Here's how the part is built. I have some questions about the finished solid (model axes, mm). A direction names the side the tool comes from. Round coordinates to 2 decimals unless told otherwise and drop trailing zeros. Order: outer loops, then holes, each group sorted by start corner. A loop starts at its lowest first (then second) coordinate and runs counter-clockwise, first axis right, second up. Notation, with made-up numbers: (41.25, -8) - (47.25, -8) arc R21 cw to (47.25, 29) - close; hole circle Ø5 at (20, 83). An arc over 180 degrees is marked (long way). Answer as a JSON object with one key per item and string values.
```python
from build123d import *

# Parameters (mm, degrees)
BOSS_EXTRUDE1_START                                 = 12.7
SKETCH1_W                                           = 108.839
SKETCH1_H                                           = 266.7
BOSS_EXTRUDE1_DEPTH                                 = 12.7
CBORE_FOR_8_BINDING_HEAD_MACHINE_SCREW1_D           = 4.9149
CBORE_FOR_8_BINDING_HEAD_MACHINE_SCREW1_CBORE_D     = 9.525
CBORE_FOR_8_BINDING_HEAD_MACHINE_SCREW1_CBORE_DEPTH = 2.667
SKETCH4_W                                           = 71.374
SKETCH4_H                                           = 223.52
CUT_EXTRUDE1_DEPTH                                  = 9.525
SKETCH6_R                                           = 2.38125
SKETCH8_W                                           = 12.7
SKETCH8_H                                           = 12.7
CUT_EXTRUDE3_DEPTH                                  = 9.525


with BuildPart() as part:
    # Sketch1 → Boss-Extrude1 (new body)
    with BuildSketch(Plane(origin=(0, 0, 0), x_dir=(1, 0, 0), z_dir=(0, 1, 0)).offset(BOSS_EXTRUDE1_START)):
        with Locations((91.6305, 133.35)):
            Rectangle(SKETCH1_W, SKETCH1_H)
    extrude(amount=BOSS_EXTRUDE1_DEPTH)

    # CBORE for #8 Binding Head Machine Screw1 (through all)
    with Locations(Plane(origin=(0, 25.4, 0), x_dir=(1, 0, 0), z_dir=(0, 1, 0))):
        with Locations((139.7, 6.35), (139.7, 260.35), (43.561, 6.35), (43.561, 260.35), (139.7, 133.35)):
            CounterBoreHole(CBORE_FOR_8_BINDING_HEAD_MACHINE_SCREW1_D / 2, CBORE_FOR_8_BINDING_HEAD_MACHINE_SCREW1_CBORE_D / 2, CBORE_FOR_8_BINDING_HEAD_MACHINE_SCREW1_CBORE_DEPTH)

    # Sketch4 → Cut-Extrude1 (cut)
    with BuildSketch(Plane(origin=(0, 12.7, 0), x_dir=(-1, 0, 0), z_dir=(0, -1, 0))):
        with Locations((-79.248, 130.175)):
            Rectangle(SKETCH4_W, SKETCH4_H)
    extrude(amount=-CUT_EXTRUDE1_DEPTH, mode=Mode.SUBTRACT)

    # Cut-Sweep1: sweep along a path in Sketch5
    with BuildLine(Plane.XZ.offset(-12.7)) as cut_sweep1_path:
        Line((114.935, -196.215), (120.015, -196.215))
        Line((120.015, -196.215), (120.015, -234.315))
        Line((120.015, -234.315), (128.905, -234.315))
        Line((128.905, -234.315), (128.905, -158.115))
        Line((128.905, -158.115), (137.795, -158.115))
        Line((137.795, -158.115), (137.795, -234.315))
        Line((137.795, -234.315), (146.05, -234.315))
    # Sketch6 → Cut-Sweep1 (sweep, cut)
    with BuildSketch(Plane(origin=(146.05, 0, 0), x_dir=(0, 0, -1), z_dir=(1, 0, 0))):
        with Locations((234.315, 12.7)):
            Circle(SKETCH6_R)
    sweep(path=cut_sweep1_path.line, transition=Transition.RIGHT, mode=Mode.SUBTRACT)

    # Sketch8 → Cut-Extrude3 (cut)
    with BuildSketch(Plane.XZ.offset(-12.7)):
        with Locations((121.285, -62.865)):
            Rectangle(SKETCH8_W, SKETCH8_H)
        with Locations((89.535, -248.285)):
            Rectangle(SKETCH8_W, SKETCH8_H)
    extrude(amount=-CUT_EXTRUDE3_DEPTH, mode=Mode.SUBTRACT)


solid = part.part
```
1. Imagine slicing it at B-B (y = 17.75). List the corners of the cut face in (x, z) for me (3 decimals), plus the area to 3 significant figures.
Responses:
{"outline": "(37.211, -266.7) - (146.05, -266.7) - (146.05, 0) - (37.211, 0) - close; hole circle Ø4.915 at (43.561, -260.35); hole circle Ø4.915 at (43.561, -6.35); hole (43.561, -241.935) - (83.185, -241.935) - (83.185, -254.635) - (95.885, -254.635) - (95.885, -241.935) - (114.935, -241.935) - (114.935, -69.215) - (127.635, -69.215) - (127.635, -56.515) - (114.935, -56.515) - (114.935, -18.415) - (43.561, -18.415) - close; hole circle Ø4.915 at (139.7, -260.35); hole circle Ø4.915 at (139.7, -133.35); hole circle Ø4.915 at (139.7, -6.35)", "area": "12,700 mm2"}
2. For faces 1 (the face through (142, 22.733, -258)), 2 (the face through (124.56, 14.92, -235.18)), 3 (the face through (142.155, 17.646, -6.458)), which set-ups out of +Z, -Z, +X, -X, +Y, -Y let a thin tool reach every point of the face, with its end or its side?
Responses:
{"face 1": "+Y", "face 2": "-Y", "face 3": "+Y, -Y"}
3. If I drill on L1, parallel to X at y = 24, z = -260.35; L2, parallel to Z at x = 139.7, y = 24.85; L3, parallel to X at y = 16.5, z = -33.5 (3 decimals), over which ranges is the centre line in solid material (lowest first)? Write a range as [from, to].
Responses:
{"L1": "[37.21, 38.8], [48.32, 134.94], [144.46, 146.05]", "L2": "[-266.7, -265.11], [-255.59, -138.11], [-128.59, -11.11], [-1.59, 0]", "L3": "[37.211, 43.561], [114.935, 146.05]"}
4. Thinking about a two-plate mould opening in Z: for faces 4 (the face through (91, 19, 0)), 5 (the face through (137.74, 15.08, -196.78)), which applies, pulls with the +Z half, pulls with the -Z half, needs draft (parallel to the pull), parting line crosses it, or undercut?
Responses:
{"face 4": "pulls with the +Z half", "face 5": "undercut"}
5. Imagine slicing it at D-D (x = 60). List the corners of the cut face in (y, z) for me (3 decimals), plus the area to 3 significant figures.
Responses:
{"outline": "(12.7, -266.7) - (25.4, -266.7) - (25.4, 0) - (12.7, 0) - (12.7, -18.415) - (22.225, -18.415) - (22.225, -241.935) - (12.7, -241.935) - close", "area": "1,260 mm2"}
6. Imagine slicing it at C-C (z = -6.35). List the corners of the cut face in (x, y) for me.
Responses:
{"outline": "(37.21, 12.7) - (41.1, 12.7) - (41.1, 22.73) - (38.8, 22.73) - (38.8, 25.4) - (37.21, 25.4) - close; (46.02, 12.7) - (137.24, 12.7) - (137.24, 22.73) - (134.94, 22.73) - (134.94, 25.4) - (48.32, 25.4) - (48.32, 22.73) - (46.02, 22.73) - close; (142.16, 12.7) - (146.05, 12.7) - (146.05, 25.4) - (144.46, 25.4) - (144.46, 22.73) - (142.16, 22.73) - close"}
7. For P1, Ø3, axis at x = 44.5, z = -262, coming from the +Y side; P2, Ø4.5, axis at x = 43.561, z = -260.35, coming from the -Y side; P3, Ø1, axis at x = 100.5, z = -125, coming from the -Y side (3 decimals), each with a flat end and sliding along its axis, tell me the tip position at first contact or that it passes through.
Responses:
{"P1": "y = 22.73", "P2": "through", "P3": "y = 22.225"}
